Check sheet for the modelled part. Datum: model origin and axes. Units: mm. A direction names the side the tool comes from. Round coordinates to 2 decimals unless told otherwise and drop trailing zeros. Order: outer loops, then holes, each group sorted by start corner. A loop starts at its lowest first (then second) coordinate and runs counter-clockwise, first axis right, second up.
from build123d import *

# Parameters (mm, degrees)
BOSS_EXTRUDE1_DEPTH = 12.7
BOSS_EXTRUDE2_DEPTH = 12.7
FILLET1_R           = 10
FILLET2_R           = 5
CHAMFER2_SIZE       = 2


with BuildPart() as part:
    # Sketch1 → Boss-Extrude1 (new body)
    with BuildSketch(Plane.XY):
        Polygon((0, 0), (-8, 0), (-8, 10), (-13, 10), (-13, -5), (5, -5), (5, 70), (10, 70), (10, 75), (0, 75), align=None)
    extrude(amount=BOSS_EXTRUDE1_DEPTH)

    # Sketch2 → Boss-Extrude2 (add)
    with BuildSketch(Plane.XY.offset(12.7)):
        Polygon((5, 10), (0, 10), (0, 0), (-8, 0), (-8, 10), (-13, 10), (-13, -5), (5, -5), align=None)
        Polygon((0, 75), (0, 70), (5, 70), (10, 70), (10, 75), align=None)
    extrude(amount=BOSS_EXTRUDE2_DEPTH)

    # Fillet1
    fillet1_edges = [part.edges().sort_by_distance(p)[0] for p in [
        (2.5, 10, 12.7),
    ]]
    fillet(fillet1_edges, radius=FILLET1_R)

    # Fillet2
    fillet2_edges = [part.edges().sort_by_distance(p)[0] for p in [
        (-13, -5, 12.7),
        (-4, -5, 25.4),
        (5, -5, 12.7),
        (-4, -5, 0),
        (10, 72.5, 0),
        (10, 72.5, 25.4),
        (2.5, 70, 12.7),
    ]]
    fillet(fillet2_edges, radius=FILLET2_R - 0.0001)  # a hair under: the kernel refuses the full size

    # Chamfer2
    chamfer2_edges = [part.edges().sort_by_distance(p)[0] for p in [
        (-13, 10, 12.7),
    ]]
    chamfer(chamfer2_edges, length=CHAMFER2_SIZE)


solid = part.part
1) Sectioned sample at A-A on y = 5.5. Record the cut outline in (x, z), and give its area (3 significant figures).
2) Set-up check for faces 1 (the face through (-9, 10, 13)), 2 (the face through (8, 73, 1)), 3 (the face through (6, 70, 15)), 4 (the face through (2, 43, 12.7)): record each of +Z, -Z, +X, -X, +Y, -Y from which the full face is reachable in a straight line by a thin tool's end or side.
3) Scan lines: line 1 (X direction, y = 3, z = 14); line 2 (X direction, y = 10.5, z = 2.5); line 3 (Y direction, x = 5.5, z = 7). Record each from-to range of solid material in increasing order.
4) Draft check along X on faces 5 (the face through (5, 35, 7)), 6 (the face through (-4, 0, 13)), 7 (the face through (-8, 5, 13)), 8 (the face through (3, 10, 24)). Enter one of: pulls with the +X half, pulls with the -X half, needs draft (parallel to the pull), parting line crosses it, or undercut.
5) Gauge pin test, flat ends, axial feed: pin 1 (12.5 mm diameter, centred on y = 40.5, z = 13.5, fed in from -X); pin 2 (12 mm diameter, centred on y = 22, z = 5, fed in from +X); pin 3 (2.5 mm diameter, centred on x = -4.5, z = 19, fed in from +Y). Record the tip position at first contact, or that the pin passes through.
6) Sectioned sample at B-B on z = 19. Record the cut outline in (x, y), and give its area (3 significant figures).
7) Sectioned sample at C-C on z = 7.25. Record the cut outline in (x, y).
Values found:
1. outline: (-13, 0) - (-8, 0) - (-8, 25.4) - (-13, 25.4) - close; (0, 0) - (5, 0) - (5, 25.4) - (0, 25.4) - close
1. area: 254 mm2
2. face 1: +Z, -Z, -X, +Y
2. face 2: -Z, +X, +Y, -Y
2. face 3: +Z, +X
2. face 4: +Z, +X, -X
3. line 1: x = -13 to -8, 0 to 5
3. line 2: x = 0 to 5
3. line 3: y = 70 to 75
4. face 5: pulls with the +X half
4. face 6: undercut
4. face 7: undercut
4. face 8: needs draft
5. pin 1: stops at x = 0
5. pin 2: stops at x = 5
5. pin 3: stops at y = 0
6. outline: (-13, 0) arc R5 ccw to (-8, -5) - (0, -5) arc R5 ccw to (5, 0) - (5, 10.71) - (0, 10.71) - (0, 0) - (-8, 0) - (-8, 10) - (-11, 10) - (-13, 8) - close; (0, 70) - (10, 70) - (10, 75) - (0, 75) - close
6. area: 231 mm2
7. outline: (-13, 0) arc R5 ccw to (-8, -5) - (0, -5) arc R5 ccw to (5, 0) - (5, 70) - (10, 70) - (10, 75) - (0, 75) - (0, 0) - (-8, 0) - (-8, 10) - (-11, 10) - (-13, 8) - close
